from build123d import *

# Parameters (mm, degrees)
F0_R      = 8.5
F1_DEPTH  = 2
F2_R      = 3.5
F3_DEPTH  = 10
F4_R      = 4
F5_DEPTH  = 4
F5_FACE_R = 4
F6_DEPTH  = 4
F6_TAPER  = -10


with BuildPart() as f1:
    # F0 (on Top) → F1 (new body)
    with BuildSketch(Plane.XY):
        Circle(F0_R)
    extrude(amount=F1_DEPTH)

    # F2 (on face) → F3 (join)
    with BuildSketch(Plane.XY.offset(2)):
        Circle(F2_R)
    extrude(amount=F3_DEPTH)

    # F4 (on face) → F5 (join)
    with BuildSketch(Plane.XY.offset(12)):
        Circle(F4_R)
    extrude(amount=F5_DEPTH)

    # F5_face (on face) → F6 (join)
    with BuildSketch(Plane.XY.offset(16)):
        Circle(F5_FACE_R)
    extrude(amount=F6_DEPTH, taper=F6_TAPER)


solid = f1.part
Here's how the part is built. I have some questions about the finished solid (model axes, mm). A direction names the side the tool comes from. Round coordinates to 2 decimals unless told otherwise and drop trailing zeros. Write each loop counter-clockwise with the first axis right and the second up, starting at its lowest first coordinate (ties: lowest second). Pieces come first, ordered by that corner, then holes. Notation, with made-up numbers: (3.25, 46) -> (33.25, 46) arc R14 cw to (33.25, 58) -> close; hole circle Ø5 at (70.25, 72). An arc over 180 degrees is marked (long way). One line per item, written item: value.
1) For faces 5 (the face through (0, 0, 0)), 6 (the face through (4, 0, 2)), which set-ups out of +Z, -Z, +X, -X, +Y, -Y let a thin tool reach every point of the face, with its end or its side?
Filled sheet:
face 5: -Z, +X, -X, +Y, -Y
face 6: none
2) Suppose I cut it at B-B on z = 8.5. List the corners of the cut face in (x, y) for me.
Filled sheet:
outline: circle Ø7 at (0, 0)
3) Suppose I cut it at D-D on x = -5.25. List the corners of the cut face in (y, z) for me, plus the area to 3 significant figures.
Filled sheet:
outline: (-6.68, 0) -> (6.68, 0) -> (6.68, 2) -> (-6.68, 2) -> close
area: 26.7 mm2
4) I'm going to push flat-ended pins straight in: pin 1 Ø1 at (x, z) = (1.5, 8) entering from +Y; pin 2 Ø2 at (x, z) = (-2, 9) entering from -Y; pin 3 Ø8 at (x, y) = (6.5, -5) entering from -Z; pin 4 Ø4 at (x, z) = (-2.5, 7.5) entering from +Y. Where does each tip first touch, or does it pass through?
Filled sheet:
pin 1: stops at y = 3.35
pin 2: stops at y = -3.35
pin 3: stops at z = 0
pin 4: stops at y = 3.46
5) Suppose I cut it at A-A on x = 0. List the corners of the cut face in (y, z) for me, plus the area to 3 significant figures.
Filled sheet:
outline: (-8.5, 0) -> (8.5, 0) -> (8.5, 2) -> (3.5, 2) -> (3.5, 12) -> (4, 12) -> (4, 16) -> (4.71, 20) -> (-4.71, 20) -> (-4, 16) -> (-4, 12) -> (-3.5, 12) -> (-3.5, 2) -> (-8.5, 2) -> close
area: 171 mm2
6) Suppose I cut it at C-C on y = -5.5. List the corners of the cut face in (x, z) for me, plus the area to 3 significant figures.
Filled sheet:
outline: (-6.48, 0) -> (6.48, 0) -> (6.48, 2) -> (-6.48, 2) -> close
area: 25.9 mm2
7) If I drill on line 1 (Z direction, x = -6.25, y = -1.25); line 2 (X direction, y = 2, z = 19.25); line 3 (X direction, y = -2.5, z = 17.25), over which ranges is the centre line in solid material (lowest first)? Write a range as [from, to].
Filled sheet:
line 1: z = [0, 2]
line 2: x = [-4.11, 4.11]
line 3: x = [-3.4, 3.4]
8) We'd pull the mould along Z, two halves only. Please class faces 1 (the face through (4.57, 7.167, 0.986)), 2 (the face through (-0.867, -3.905, 13.972)), 3 (the face through (3.233, -1.341, 6.93)), 4 (the face through (0, 0, 20)): released by +Z, released by -Z, zero draft, split by the parting line, or undercut.
Filled sheet:
face 1: zero draft
face 2: undercut
face 3: undercut
face 4: released by +Z
